Work out the finished part from the listing and answer in its coordinate system (mm). Face numbers are marked on the shaded views. A direction names the side the tool comes from. Give positions to 0.01 mm unless a question says otherwise; leave off trailing zeros. Write each loop counter-clockwise with the first axis right and the second up, starting at its lowest first coordinate (ties: lowest second). Pieces come first, ordered by that corner, then holes.
1) Straight lines are drawn through the part: probe 1 along Y at (x, z) = (67.1, 5.5); probe 2 along Y at (x, z) = (24, 4); probe 3 along Y at (x, z) = (-19.07, 7.15). For each, find the intervals that lie inside material, in ascending order.
2) Find section B-B (z = 2.5). Determine the outline of the cut face in (x, y), plus the area to 3 significant figures.
3) Determine the mould class of the marked faces 1, 2, 3 and 4 for opening direction X: pulls with the +X half, pulls with the -X half, needs draft (parallel to the pull), parting line crosses it, or undercut.
4) Find section A-A (x = -19.07). Determine the outline of the cut face in (y, z).
5) Find section D-D (y = 0). Count the separate pieces of the cut face and the enclosed holes in it, plus the area to 3 significant figures.
6) A tool of negligible diameter and unlimited length cuts with its end or side. For the marked faces 5, 6 and 7, from which of +Z, -Z, +X, -X, +Y, -Y can it reach the whole face along a straight path? Write none if from no direction.
7) Find section C-C (x = 1). Determine the outline of the cut face in (y, z), plus the area to 3 significant figures.
8) Given pin 1 Ø3 at (x, y) = (16, -13.5) entering from -Z; pin 2 Ø6.5 at (x, y) = (67.1, 0) entering from -Z; pin 3 Ø8 at (x, y) = (19.07, 0) entering from +Z; pin 4 Ø3 at (x, y) = (-31.5, 1) entering from -Z, each flat-ended and moving along its own axis, determine where each tip first touches the part or whether it passes through.
```python
from build123d import *

# Parameters (mm, degrees)
SKETCH_1_W          = 114
SKETCH_1_H          = 56
SKETCH_1_W_2        = 110
SKETCH_1_H_2        = 52
EXTRUDE_1_DEPTH     = 7
SKETCH_2_W          = 114
SKETCH_2_H          = 56
EXTRUDE_1_2_DEPTH   = 1.2
SKETCH_3_R          = 2.5
CUT_EXTRUDE_1_DEPTH = 1.2
FILLET_1_R          = 20
FILLET_2_R          = 21
SKETCH_4_W          = 33.86
SKETCH_4_H          = 14
EXTRUDE_2_DEPTH     = 1.2
SKETCH_5_R          = 2.5
CUT_EXTRUDE_2_DEPTH = 1.2
FILLET_3_R          = 0.1
SKETCH_6_W          = 25
SKETCH_6_H          = 22.2
EXTRUDE_3_DEPTH     = 7
CUT_EXTRUDE_3_DEPTH = 0.4
SKETCH_8_W          = 27
SKETCH_8_H          = 18.2
CUT_EXTRUDE_4_DEPTH = 5
SKETCH_11_W         = 2
SKETCH_11_H         = 27
EXTRUDE_4_DEPTH     = 8.2
SKETCH_12_W         = 2
SKETCH_12_H         = 18.2
CUT_EXTRUDE_5_DEPTH = 5
SKETCH_13_R         = 2.5
SKETCH_13_R_2       = 2
CUT_EXTRUDE_6_DEPTH = 7


with BuildPart() as part:
    # Эскиз1 → Extrude 1 (new body)
    with BuildSketch(Plane.XY):
        Rectangle(SKETCH_1_W, SKETCH_1_H)
        Rectangle(SKETCH_1_W_2, SKETCH_1_H_2, mode=Mode.SUBTRACT)
    extrude(amount=EXTRUDE_1_DEPTH)

    # Эскиз2 → Extrude 1 2 (add)
    with BuildSketch(Plane.XY.offset(7)):
        Rectangle(SKETCH_2_W, SKETCH_2_H)
    extrude(amount=EXTRUDE_1_2_DEPTH)

    # Эскиз3 → Вырез-Вытянуть1 (cut)
    with BuildSketch(Plane.XY.offset(8.2)):
        with Locations((-38.93, 0)):
            Circle(SKETCH_3_R)
        with Locations((-29, 0)):
            Circle(SKETCH_3_R)
        with Locations((-19.07, 0)):
            Circle(SKETCH_3_R)
        with Locations((19.07, 0)):
            Circle(SKETCH_3_R)
        with Locations((29, 0)):
            Circle(SKETCH_3_R)
        with Locations((38.93, 0)):
            Circle(SKETCH_3_R)
    extrude(amount=-CUT_EXTRUDE_1_DEPTH, mode=Mode.SUBTRACT)

    # Скругление1
    fillet_1_edges = [part.edges().sort_by_distance(p)[0] for p in [
        (-55, 26, 3.5),
        (-55, -26, 3.5),
        (55, -26, 3.5),
        (55, 26, 3.5),
    ]]
    fillet(fillet_1_edges, radius=FILLET_1_R)

    # Скругление2
    fillet_2_edges = [part.edges().sort_by_distance(p)[0] for p in [
        (-57, 28, 4.1),
        (57, 28, 4.1),
        (57, -28, 4.1),
        (-57, -28, 4.1),
    ]]
    fillet(fillet_2_edges, radius=FILLET_2_R)

    # Эскиз4 → Бобышка-Вытянуть2 (add)
    with BuildSketch(Plane(origin=(0, 0, 7), x_dir=(-1, 0, 0), z_dir=(0, 0, -1))):
        with Locations((29, 0)):
            Rectangle(SKETCH_4_W, SKETCH_4_H)
        with Locations((-29, 0)):
            Rectangle(SKETCH_4_W, SKETCH_4_H)
    extrude(amount=EXTRUDE_2_DEPTH)

    # Эскиз5 → Вырез-Вытянуть2 (cut)
    with BuildSketch(Plane.XY.offset(7)):
        with Locations((-29, 0)):
            Circle(SKETCH_5_R)
        with Locations((-38.93, 0)):
            Circle(SKETCH_5_R)
        with Locations((-19.07, 0)):
            Circle(SKETCH_5_R)
        with Locations((19.07, 0)):
            Circle(SKETCH_5_R)
        with Locations((29, 0)):
            Circle(SKETCH_5_R)
        with Locations((38.93, 0)):
            Circle(SKETCH_5_R)
    extrude(amount=-CUT_EXTRUDE_2_DEPTH, mode=Mode.SUBTRACT)

    # Скругление3
    fillet_3_edges = [part.edges().sort_by_distance(p)[0] for p in [
        (36.43, 0, 5.8),
        (16.57, 0, 5.8),
        (-21.57, 0, 5.8),
        (-41.43, 0, 5.8),
    ]]
    fillet(fillet_3_edges, radius=FILLET_3_R)

    # Эскиз6 → Бобышка-Вытянуть3 (add)
    with BuildSketch(Plane(origin=(0, 0, 7), x_dir=(-1, 0, 0), z_dir=(0, 0, -1))):
        with Locations((-67.5, 1.5)):
            Rectangle(SKETCH_6_W, SKETCH_6_H)
    extrude(amount=EXTRUDE_3_DEPTH)

    # Эскиз7 → Вырез-Вытянуть3 (cut)
    with BuildSketch(Plane.XY.offset(7)):
        with BuildLine():
            Line((57, 7), (57, -7))
            ThreePointArc((57, -7), (56.959567588, -8.302507787), (56.838426044, -9.6))
            Line((56.838426044, -9.6), (80, -9.6))
            Line((80, -9.6), (80, 12.6))
            Line((80, 12.6), (56.239565213, 12.6))
            ThreePointArc((56.239565213, 12.6), (56.809022916, 9.825697306), (57, 7))
        make_face()
    extrude(amount=-CUT_EXTRUDE_3_DEPTH, mode=Mode.SUBTRACT)

    # Эскиз8 → Вырез-Вытянуть4 (cut)
    with BuildSketch(Plane(origin=(0, 0, 0), x_dir=(-1, 0, 0), z_dir=(0, 0, -1))):
        with Locations((-66.5, 1.5)):
            Rectangle(SKETCH_8_W, SKETCH_8_H)
    extrude(amount=-CUT_EXTRUDE_4_DEPTH, mode=Mode.SUBTRACT)

    # Эскиз11 → Бобышка-Вытянуть4 (add)
    with BuildSketch(Plane.XY.offset(8.2)):
        with Locations((56, 1.5)):
            Rectangle(SKETCH_11_W, SKETCH_11_H)
    extrude(amount=-EXTRUDE_4_DEPTH)

    # Эскиз12 → Вырез-Вытянуть5 (cut)
    with BuildSketch(Plane(origin=(0, 0, 0), x_dir=(-1, 0, 0), z_dir=(0, 0, -1))):
        with Locations((-56, 1.5)):
            Rectangle(SKETCH_12_W, SKETCH_12_H)
    extrude(amount=-CUT_EXTRUDE_5_DEPTH, mode=Mode.SUBTRACT)

    # Эскиз13 → Вырез-Вытянуть6 (cut)
    with BuildSketch(Plane(origin=(0, 0, 5), x_dir=(-1, 0, 0), z_dir=(0, 0, -1))):
        with Locations((-67.1, 0)):
            Circle(SKETCH_13_R)
        with Locations((-67.210919407, 6)):
            Circle(SKETCH_13_R_2)
    extrude(amount=-CUT_EXTRUDE_6_DEPTH, mode=Mode.SUBTRACT)


solid = part.part
```
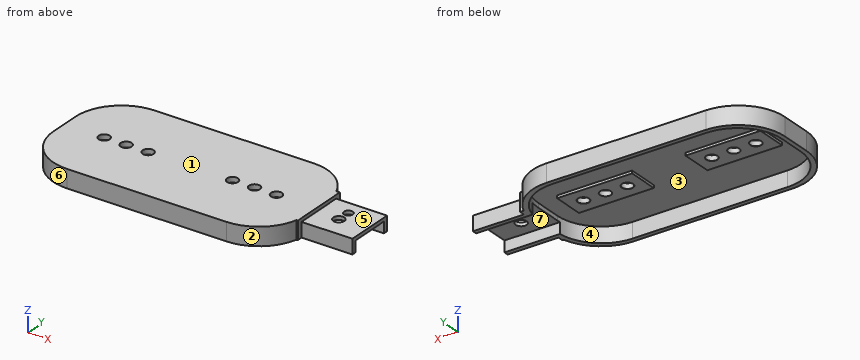
Results:
1. probe 1: y = -9.6 to -2.5, 2.5 to 4, 8 to 12.6
1. probe 2: y = -28 to -26, 26 to 28
1. probe 3: y = -28 to -2.5, 2.5 to 28
2. outline: (-57, -7) arc R21 ccw to (-36, -28) - (36, -28) arc R21 ccw to (56.4, -12) - (57, -12) - (57, -9.6) - (80, -9.6) - (80, -7.6) - (54.94, -7.6) arc R20 cw to (35, -26) - (-35, -26) arc R20 cw to (-55, -6) - (-55, 6) arc R20 cw to (-35, 26) - (35, 26) arc R20 cw to (54.46, 10.6) - (80, 10.6) - (80, 12.6) - (57, 12.6) - (57, 15) - (55.42, 15) arc R21 ccw to (36, 28) - (-36, 28) arc R21 ccw to (-57, 7) - close
2. area: 689 mm2
3. face 1: needs draft
3. face 2: pulls with the +X half
3. face 3: undercut
3. face 4: undercut
4. outline: (-28, 0) - (-26, 0) - (-26, 7) - (-7, 7) - (-7, 5.8) - (-2.6, 5.8) arc R0.1 ccw to (-2.5, 5.9) - (-2.5, 8.2) - (-28, 8.2) - close; (2.5, 5.9) arc R0.1 ccw to (2.6, 5.8) - (7, 5.8) - (7, 7) - (26, 7) - (26, 0) - (28, 0) - (28, 8.2) - (2.5, 8.2) - close
5. separate pieces: 8
5. enclosed holes: 0
5. area: 193 mm2
6. face 5: +Z, +X, +Y, -Y
6. face 6: +Z, -Z, -X, -Y
6. face 7: -Z, +X
7. outline: (-28, 0) - (-26, 0) - (-26, 7) - (26, 7) - (26, 0) - (28, 0) - (28, 8.2) - (-28, 8.2) - close
7. area: 95.2 mm2
8. pin 1: stops at z = 7
8. pin 2: stops at z = 5
8. pin 3: stops at z = 8.2
8. pin 4: stops at z = 5.8
